Read the model definition and answer for the solid it produces. Units are mm, in the model's axes. Face numbers are marked on the shaded views. A direction names the side the tool comes from. Give positions to 0.01 mm unless a question says otherwise; leave off trailing zeros. Loops run counter-clockwise (first coordinate to the right, second up) from the corner with the lowest first, then second, coordinate; pieces in that order, holes last.
(1) Find section C-C, the plane x = -26.5. Write down the section's boundary in (y, z) (3 decimals).
(2) Straight lines are drawn through the part: probe 1 along Y at (x, z) = (-45, 198.5) (3 decimals); probe 2 along X at (y, z) = (5, 146) (3 decimals); probe 3 along X at (y, z) = (11, 44) (3 decimals). For each, find the intervals that lie inside material, in ascending order.
(3) Which of the six approach directions +Z, -Z, +X, -X, +Y, -Y give full straight-line access (tool end or side, diameter ignored) to the marked faces 1 and 2?
(4) Determine the mould class of the marked faces 3, 4, 5 and 6 for opening direction X: pulls with the +X half, pulls with the -X half, needs draft (parallel to the pull), parting line crosses it, or undercut.
(5) Find section B-B, the plane z = 164. Write down the section's boundary in (x, y) (3 decimals).
(6) This flat-tipped pin is pushed along its axis until it touches: P1, Ø8, axis at x = -10, y = 21, coming from the -Z side. Where does it stop, or does it pass through?
(7) Find section A-A, the plane y = 5.25. Write down the section's boundary in (x, z) (3 decimals).
(8) Find section D-D, the plane z = 22.5. Write down the section's boundary in (x, y) (3 decimals).
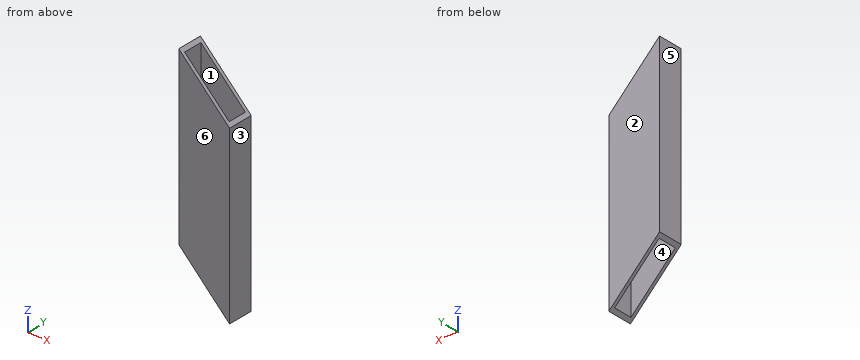
```python
from build123d import *

# Parameters (mm, degrees)
F0_W     = 50.8
F0_H     = 25.4
F0_W_2   = 44.45
F0_H_2   = 19.05
F1_DEPTH = 222.77578
F3_DEPTH = 25.4


with BuildPart() as f1:
    # F0 (on Top) → F1 (new body)
    with BuildSketch(Plane.XY):
        with Locations((-25.4, 12.7)):
            Rectangle(F0_W, F0_H)
        with Locations((-25.4, 12.7)):
            Rectangle(F0_W_2, F0_H_2, mode=Mode.SUBTRACT)
    extrude(amount=F1_DEPTH)

    # F2 (on face) → F3 (cut)
    with BuildSketch(Plane.XZ):
        Polygon((-50.8, 0), (0, 0), (-50.8, 50.8), align=None)
        Polygon((-50.8, 222.77578), (0, 171.97578), (0, 222.77578), align=None)
    extrude(amount=-F3_DEPTH, mode=Mode.SUBTRACT)


solid = f1.part
```
Entries:
1. outline: (0, 26.5) - (3.175, 26.5) - (3.175, 198.476) - (0, 198.476) - close; (22.225, 26.5) - (25.4, 26.5) - (25.4, 198.476) - (22.225, 198.476) - close
2. probe 1: y = 0 to 3.175, 22.225 to 25.4
2. probe 2: x = -50.8 to -47.625, -3.175 to 0
2. probe 3: x = -3.175 to 0
3. face 1: +Z, -Z
3. face 2: +Z, -Z, +X, -X, +Y
4. face 3: pulls with the +X half
4. face 4: undercut
4. face 5: pulls with the -X half
4. face 6: needs draft
5. outline: (-50.8, 0) - (0, 0) - (0, 25.4) - (-50.8, 25.4) - close; hole (-47.625, 3.175) - (-3.175, 3.175) - (-3.175, 22.225) - (-47.625, 22.225) - close
6. P1: stops at z = 6.19
7. outline: (-50.8, 50.8) - (-47.625, 47.625) - (-47.625, 219.601) - (-50.8, 222.776) - close; (-3.175, 3.175) - (0, 0) - (0, 171.976) - (-3.175, 175.151) - close
8. outline: (-22.5, 0) - (0, 0) - (0, 25.4) - (-22.5, 25.4) - (-22.5, 22.225) - (-3.175, 22.225) - (-3.175, 3.175) - (-22.5, 3.175) - close
